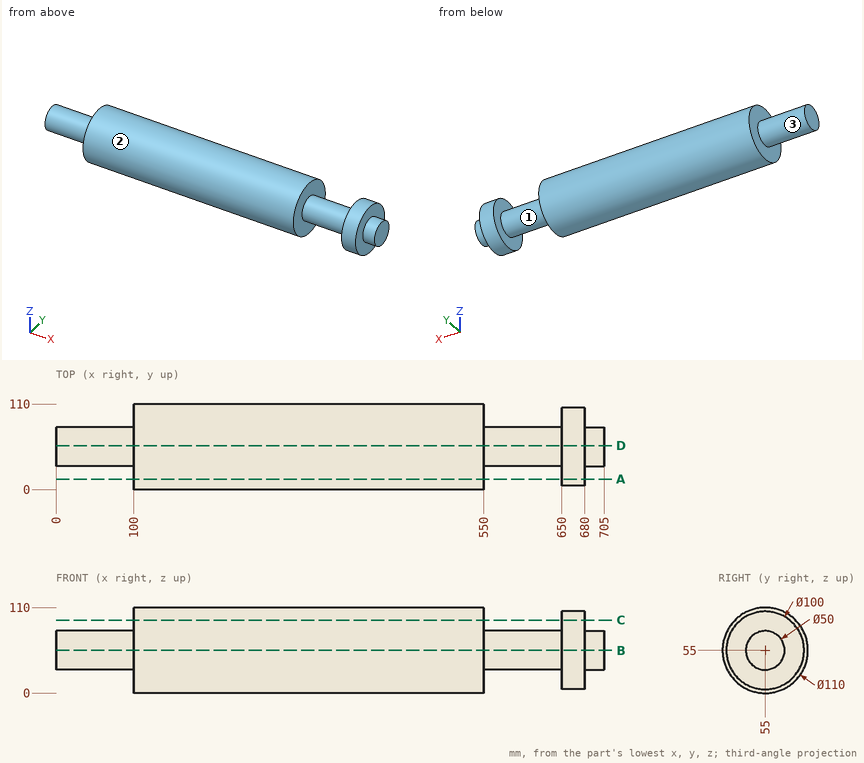
Geometry: see drawing. Coordinates: mm, zero at the bounding-box minimum. A direction names the side the tool comes from. Coordinates: 2 decimals unless noted, no trailing zeros. Write each loop counter-clockwise with the first axis right and the second up, starting at its lowest first coordinate (ties: lowest second). Pieces come first, ordered by that corner, then holes.
1) Section B-B on z = 55. Output: boundary loops of the cut face in (x, y).
2) Section A-A on y = 13.5. Output: boundary loops of the cut face in (x, z).
3) Set-up query: the marked faces 1, 2 and 3. Return all of +Z, -Z, +X, -X, +Y, -Y with unobstructed straight access to the full face (end or side cutting, diameter ignored); none if empty.
4) Material intervals for line 1 along X through (y, z) = (44.5, 7.5); line 2 along X through (y, z) = (101.5, 78); line 3 along Z through (x, y) = (502.5, 58), sorted ascending.
5) Section C-C on z = 94. Output: boundary loops of the cut face in (x, y).
6) Section D-D on y = 56.5. Output: boundary loops of the cut face in (x, z), and give its area (3 significant figures).
7) Pin query (flat end, axial travel): pin 1 Ø10 at (x, z) = (147, 61) entering from -Y; pin 2 Ø2 at (x, y) = (490, 77) entering from -Z; pin 3 Ø4 at (x, z) = (517, 78.5) entering from +Y. Return the tip coordinate at first contact, or that it passes through.
Check result:
1. outline: (0, 30) - (100, 30) - (100, 0) - (550, 0) - (550, 30) - (650, 30) - (650, 5) - (680, 5) - (680, 30) - (705, 30) - (705, 80) - (680, 80) - (680, 105) - (650, 105) - (650, 80) - (550, 80) - (550, 110) - (100, 110) - (100, 80) - (0, 80) - close
2. outline: (100, 18.91) - (550, 18.91) - (550, 91.09) - (100, 91.09) - close; (650, 27.11) - (680, 27.11) - (680, 82.89) - (650, 82.89) - close
3. face 1: none
3. face 2: +X, -X
3. face 3: -X
4. line 1: x = 100 to 550, 650 to 680
4. line 2: x = 100 to 550
4. line 3: z = 0.08 to 109.92
5. outline: (100, 16.22) - (550, 16.22) - (550, 93.78) - (100, 93.78) - close; (650, 23.71) - (680, 23.71) - (680, 86.29) - (650, 86.29) - close
6. outline: (0, 30.05) - (100, 30.05) - (100, 0.02) - (550, 0.02) - (550, 30.05) - (650, 30.05) - (650, 5.02) - (680, 5.02) - (680, 30.05) - (705, 30.05) - (705, 79.95) - (680, 79.95) - (680, 104.98) - (650, 104.98) - (650, 79.95) - (550, 79.95) - (550, 109.98) - (100, 109.98) - (100, 79.95) - (0, 79.95) - close
6. area: 63,700 mm2
7. pin 1: stops at y = 0.01
7. pin 2: stops at z = 4.17
7. pin 3: stops at y = 105.62
